Can you work these out from the model? Positions are in its coordinate system, mm. Face numbers are marked on the shaded views. A direction names the side the tool comes from. Coordinates: 2 decimals unless noted, no trailing zeros. Order: outer loops, then holes, each group sorted by start corner. A loop starts at its lowest first (then second) coordinate and runs counter-clockwise, first axis right, second up. Notation, with made-up numbers: (-39.5, 17.5) -> (-34.5, 17.5) arc R17 ccw to (-34.5, 29.5) -> close; hole circle Ø2 at (-32, -12.5). An arc over 180 degrees is marked (long way). Answer in a Markdown table with one row per item. Add a question column.
1. Imagine slicing it at A-A on z = -17. Write out the boundary of the cut face in (x, y), plus the area to 3 significant figures.
2. If I drill on line 1 along Z through (x, y) = (8, 5); line 2 along Z through (x, y) = (17, -7); line 3 along Z through (x, y) = (-13.5, 18), over which ranges is the centre line in solid material (lowest first)? Write a range as [from, to].
3. Imagine slicing it at B-B on y = -8.5. State how many separate pieces and enclosed holes the cut face has, plus the area to 4 significant figures.
4. Imagine slicing it at D-D on z = 10. Write out the boundary of the cut face in (x, y), plus the area to 3 significant figures.
5. On a 3-axis mill with a long thin cutter (end or side, diameter ignored), from which of +Z, -Z, +X, -X, +Y, -Y can I reach the whole of each face in a straight line? I mean the marked faces 5 and 6. Say none if no direction works.
6. Will these pins go through, and if not, where does the flat tip stop? pin 1 (5 mm diameter, centred on x = 4.5, z = -35.5, fed in from -Y); pin 2 (1.5 mm diameter, centred on x = 6.5, z = 35, fed in from -Y); pin 3 (10 mm diameter, centred on x = 6.5, y = 8, fed in from +Z); pin 4 (4 mm diameter, centred on x = -17.5, z = 10.5, fed in from -Y) (3 decimals).
7. We'd pull the mould along X, two halves only. Please class the marked faces 1, 2, 3 and 4: pulls with the +X half, pulls with the -X half, needs draft (parallel to the pull), parting line crosses it, or undercut.
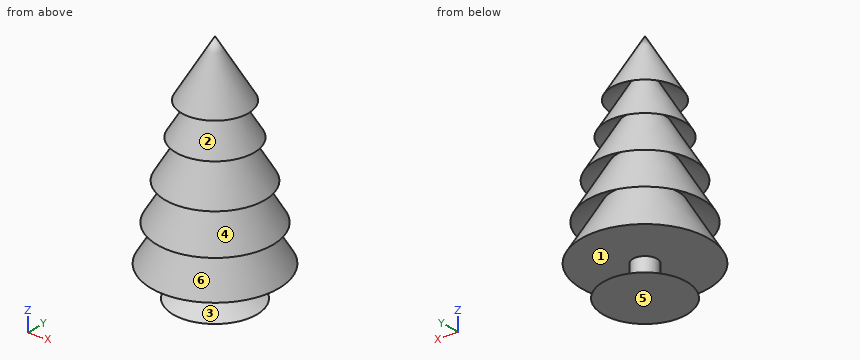
from build123d import *

# Parameters (mm, degrees)
F0_W = 5.6183873676
F0_H = 8.2852373922


with BuildPart() as f1:
    # F0 (on Front) → F1 (revolve)
    with BuildSketch(Plane.XZ):
        Polygon((15.6066315249, 28.4040719271), (0, 54.8312999308), (0, -38.8467890119), (5.6183873676, -38.8467890119), (29.8360655374, -38.8467890119), (15.6066315249, -14.7516153408), (27.0295340755, -21.8909281701), (13.1205966132, 1.6615380376), (23.3266572773, -4.7172487474), (9.5442305374, 18.6209926483), (18.3223614144, 13.1346618221), (5.6183873676, 34.6467234194), align=None)
        with Locations((2.8091936838, -42.989407708)):
            Rectangle(F0_W, F0_H)
        Polygon((5.6183873676, -47.1320264041), (0, -47.1320264041), (0, -53.1665943563), (19.5603128523, -53.1665943563), align=None)
    revolve(axis=Axis((0, 0, 7.9922554594), (0, 0, 1)))


solid = f1.part
Answers follow:
| question | item | result |
|---|---|---|
| 1 | outline | circle Ø48.28 at (0, 0); circle Ø33.87 at (0, 0); hole circle Ø38.41 at (0, 0) |
| 1 | area | 1,570 mm² |
| 2 | line 1 | z = [-53.17, -48.78], [-38.85, 28.19], [32.26, 38.86] |
| 2 | line 2 | z = [-53.17, -52.66], [-38.85, -19.46], [-16.49, -7.25], [-1.63, 3.65] |
| 2 | line 3 | z = [-38.85, -26.42], [-19.06, -14.22], [-4.2, -3.32] |
| 3 | separate pieces | 3 |
| 3 | enclosed holes | 0 |
| 3 | area | 2,465 mm² |
| 4 | outline | circle Ø29.27 at (0, 0) |
| 4 | area | 673 mm² |
| 5 | face 5 | -Z, +X, -X, +Y, -Y |
| 5 | face 6 | none |
| 6 | pin 1 | stops at y = -29.03 |
| 6 | pin 2 | stops at y = -10.44 |
| 6 | pin 3 | stops at z = 45.84 |
| 6 | pin 4 | passes through |
| 7 | face 1 | needs draft |
| 7 | face 2 | undercut |
| 7 | face 3 | parting line crosses it |
| 7 | face 4 | undercut |
